Read the model definition and answer for the solid it produces. Units are mm, in the model's axes. A direction names the side the tool comes from. Coordinates: 2 decimals unless noted, no trailing zeros. Write each loop counter-clockwise with the first axis right and the second up, starting at its lowest first coordinate (ties: lowest second). Pieces come first, ordered by that corner, then holes. Notation, with made-up numbers: (9.25, -21) - (31.25, -21) arc R14 cw to (31.25, -2) - close; hole circle Ø9 at (60, 8). An arc over 180 degrees is marked (long way). Return JSON: item names as keys, results as strings.
```python
from build123d import *

# Parameters (mm, degrees)
F0_W     = 13.951736
F0_H     = 20.6375
F0_W_2   = 83.132682
F1_DEPTH = 50.8
F2_W     = 129.48776
F2_H     = 20.6375
F3_DEPTH = 50.8


with BuildPart() as f1:
    # F0 (on Top) → F1 (new body)
    with BuildSketch(Plane.XY):
        Polygon((-150.996204, 0), (-31.4737, 0), (31.4737, 0), (31.4737, 20.6375), (-22.181449, 20.6375), (-146.704241, 20.6375), (-150.996204, 20.6375), align=None)
        Polygon((31.4737, 0), (-31.4737, 0), (-31.4737, -20.6375), (22.181449, -20.6375), (146.704241, -20.6375), (150.996204, -20.6375), (150.996204, 0), align=None)
        Polygon((-31.4737, -20.6375), (-31.4737, 0), (-150.996204, 0), (-150.996204, -20.6375), (-146.704241, -20.6375), align=None)
        Polygon((31.4737, 20.6375), (31.4737, 0), (150.996204, 0), (150.996204, 20.6375), (146.704241, 20.6375), align=None)
        Polygon((22.181449, -20.6375), (-31.4737, -20.6375), (-146.704241, -20.6375), (-146.704241, -41.275), (-139.257324, -41.275), (-70.105411, -41.275), (22.181449, -41.275), align=None)
        Polygon((-22.181449, 20.6375), (31.4737, 20.6375), (146.704241, 20.6375), (146.704241, 41.275), (139.257324, 41.275), (70.105411, 41.275), (-22.181449, 41.275), align=None)
        Polygon((146.704241, -20.6375), (22.181449, -20.6375), (22.181449, -41.275), (139.257324, -41.275), (146.704241, -41.275), align=None)
        Polygon((-146.704241, 20.6375), (-22.181449, 20.6375), (-22.181449, 41.275), (-139.257324, 41.275), (-146.704241, 41.275), align=None)
        Polygon((139.257324, -41.275), (22.181449, -41.275), (-70.105411, -41.275), (-70.105411, -61.9125), (-32.869801, -61.9125), (96.617959, -61.9125), (128.10643, -61.9125), (139.257324, -61.9125), align=None)
        Polygon((-139.257324, 41.275), (-22.181449, 41.275), (70.105411, 41.275), (70.105411, 61.9125), (32.869801, 61.9125), (-96.617959, 61.9125), (-128.10643, 61.9125), (-139.257324, 61.9125), align=None)
        Polygon((-70.105411, -61.9125), (-70.105411, -41.275), (-139.257324, -41.275), (-139.257324, -61.9125), (-128.10643, -61.9125), align=None)
        Polygon((70.105411, 41.275), (139.257324, 41.275), (139.257324, 61.9125), (128.10643, 61.9125), (70.105411, 61.9125), align=None)
        Polygon((-32.869801, -61.9125), (-70.105411, -61.9125), (-128.10643, -61.9125), (-128.10643, -82.55), (-112.152128, -82.55), (-32.869801, -82.55), align=None)
        Polygon((32.869801, 61.9125), (70.105411, 61.9125), (128.10643, 61.9125), (128.10643, 82.55), (112.152128, 82.55), (32.869801, 82.55), align=None)
        Polygon((128.10643, -82.55), (128.10643, -61.9125), (96.617959, -61.9125), (96.617959, -82.55), (112.152128, -82.55), align=None)
        Polygon((-128.10643, 82.55), (-128.10643, 61.9125), (-96.617959, 61.9125), (-96.617959, 82.55), (-112.152128, 82.55), align=None)
        Polygon((55.90756, -82.55), (-32.869801, -82.55), (-112.152128, -82.55), (-112.152128, -103.1875), (-88.843285, -103.1875), (55.90756, -103.1875), align=None)
        Polygon((-55.90756, 82.55), (32.869801, 82.55), (112.152128, 82.55), (112.152128, 103.1875), (88.843285, 103.1875), (-55.90756, 103.1875), align=None)
        Polygon((112.152128, -82.55), (96.617959, -82.55), (55.90756, -82.55), (55.90756, -103.1875), (88.843285, -103.1875), (112.152128, -103.1875), align=None)
        Polygon((-112.152128, 82.55), (-96.617959, 82.55), (-55.90756, 82.55), (-55.90756, 103.1875), (-88.843285, 103.1875), (-112.152128, 103.1875), align=None)
        Polygon((88.843285, -103.1875), (55.90756, -103.1875), (-88.843285, -103.1875), (-88.843285, -123.825), (-48.542209, -123.825), (34.590473, -123.825), (48.542209, -123.825), (88.843285, -123.825), align=None)
        Polygon((-88.843285, 103.1875), (-55.90756, 103.1875), (88.843285, 103.1875), (88.843285, 123.825), (48.542209, 123.825), (-34.590473, 123.825), (-48.542209, 123.825), (-88.843285, 123.825), align=None)
        with Locations((41.566341, -134.14375)):
            Rectangle(F0_W, F0_H)
        with Locations((-6.975868, -134.14375)):
            Rectangle(F0_W_2, F0_H)
        with Locations((6.975868, 134.14375)):
            Rectangle(F0_W_2, F0_H)
        with Locations((-41.566341, 134.14375)):
            Rectangle(F0_W, F0_H)
    extrude(amount=F1_DEPTH)

    # F2 (on face) → F3 (join)
    with BuildSketch(Plane.XY.offset(50.8)):
        with Locations((31.874079, -72.23125)):
            Rectangle(F2_W, F2_H)
        with Locations((-31.874079, 72.23125)):
            Rectangle(F2_W, F2_H)
    extrude(amount=-F3_DEPTH)


solid = f1.part
```
(1) Determine the mould class of faces 1 (the face through (112.152, 93, 25)), 2 (the face through (-128.106, -72, 25)), 3 (the face through (-69, -123.825, 25)) for opening direction X: +X half, -X half, draft (parallel to the pull), parting line (faces both ways), or undercut.
Answer:
{"face 1": "+X half", "face 2": "-X half", "face 3": "draft"}
(2) A cutting plane is placed at A-A (y = 46). Determine the outline of the cut face in (x, z).
Answer:
{"outline": "(-139.26, 0) - (139.26, 0) - (139.26, 50.8) - (-139.26, 50.8) - close"}
(3) A cutting plane is placed at B-B (x = 66). Determine the outline of the cut face in (y, z) (3 decimals).
Answer:
{"outline": "(-123.825, 0) - (123.825, 0) - (123.825, 50.8) - (-123.825, 50.8) - close"}
(4) Which of the six approach directions +Z, -Z, +X, -X, +Y, -Y give full straight-line access (tool end or side, diameter ignored) to faces 4 (the face through (134, -61.912, 25)), 5 (the face through (-100, 103.188, 25)), 6 (the face through (88.843, 113, 25)), 7 (the face through (-146.704, -31, 25))?
Answer:
{"face 4": "+Z, -Z, +X, -Y", "face 5": "+Z, -Z, -X, +Y", "face 6": "+Z, -Z, +X, +Y", "face 7": "+Z, -Z, -X, -Y"}
(5) Flat-ended cylindrical pins translate along their axes: P1, Ø12, axis at y = 30, z = 12, coming from the -X side; P2, Ø10.5, axis at y = -49, z = 14.5, coming from the -X side; P3, Ø4.5, axis at x = 149.5, z = 38, coming from the -Y side; P4, Ø16.5, axis at y = -28.5, z = 34.5, coming from the -X side. Find the tip coordinate at first contact, or state that the pin passes through.
Answer:
{"P1": "x = -146.7", "P2": "x = -139.26", "P3": "y = -20.64", "P4": "x = -151"}
(6) Straight lines are drawn through the part: line 1 (Y direction, x = 70.5, z = 29) (3 decimals); line 2 (X direction, y = -46, z = 36.5); line 3 (X direction, y = 30, z = 37). For each, find the intervals that lie inside material, in ascending order. Write a range as from..to.
Answer:
{"line 1": "-123.825..123.825", "line 2": "-139.26..139.26", "line 3": "-146.7..146.7"}
